from build123d import *

# Parameters (mm, degrees)
BOSS_EXTRUDE1_DEPTH       = 1.5875
F_4_CLEARANCE_HOLE1_D     = 2.9464
F_4_CLEARANCE_HOLE1_DEPTH = 3.302
F_4_CLEARANCE_HOLE1_TIP   = 0.885187864
SKETCH5_W                 = 1.7399
SKETCH5_H                 = 25.4
BOSS_EXTRUDE2_DEPTH       = 1.5875


with BuildPart() as part:
    # Sketch1 → Boss-Extrude1 (new body)
    with BuildSketch(Plane.XY):
        with BuildLine():
            Line((3.58902, 12.7), (3.58902, -12.7))
            ThreePointArc((3.58902, -12.7), (0, -16.28902), (-3.58902, -12.7))
            Line((-3.58902, -12.7), (-3.58902, 12.7))
            ThreePointArc((-3.58902, 12.7), (0, 16.28902), (3.58902, 12.7))
        make_face()
    extrude(amount=BOSS_EXTRUDE1_DEPTH)

    # #4 Clearance Hole1
    with Locations(Plane.XY.offset(1.5875)):
        with Locations((0, 12.7), (0, -12.7)):
            Hole(F_4_CLEARANCE_HOLE1_D / 2, depth=F_4_CLEARANCE_HOLE1_DEPTH)
            with Locations((0, 0, -(F_4_CLEARANCE_HOLE1_DEPTH + F_4_CLEARANCE_HOLE1_TIP / 2))):  # 118° drill point
                Cone(0, F_4_CLEARANCE_HOLE1_D / 2, F_4_CLEARANCE_HOLE1_TIP, mode=Mode.SUBTRACT)

    # Sketch5 → Boss-Extrude2 (add)
    with BuildSketch(Plane.XY.offset(1.5875)):
        with Locations((4.45897, 0)):
            Rectangle(SKETCH5_W, SKETCH5_H)
    extrude(amount=-BOSS_EXTRUDE2_DEPTH)


solid = part.part
For this review, take the finished solid that the model builds, in its own axes (mm). A direction names the side the tool comes from. Round coordinates to 2 decimals unless told otherwise and drop trailing zeros. Order: outer loops, then holes, each group sorted by start corner. A loop starts at its lowest first (then second) coordinate and runs counter-clockwise, first axis right, second up. Notation, with made-up numbers: M 76,-28 L 85,-28 A20 ccw 85,-21 Z; hole C 34.25,71 d3. An arc over 180 degrees is marked long. Write each question's results on one line, items separated by ' | '. Start each with the question number.
1. Clearance check with a flat-ended pin moving along its axis: pin 1 Ø0.8 at (x, z) = (4.5, 1) entering from +Y. State where the tip first meets the part, or that it passes through.
2. Add section B-B (z = 0.45). State the section outline as (x, y) points, then the cut area to 3 significant figures.
3. Add section A-A (x = 0). State the section outline as (y, z) points.
4. Add section C-C (y = 11.5). State the section outline as (x, z) points.
5. Draft analysis for pull direction Y (two halves, no side actions). For faces 3 (the face through (0.19, -11.24, 0.78)), 4 (the face through (4, 12.7, 1)), 5 (the face through (0.08, -16.29, 0.78)), state which applies: pulls with the +Y half, pulls with the -Y half, needs draft (parallel to the pull), parting line crosses it, or undercut.
6. Tool access review of faces 1 (the face through (4, -12.7, 1)), 2 (the face through (-0.08, 16.29, 0.78)): name each direction out of +Z, -Z, +X, -X, +Y, -Y from which nothing blocks a thin tool from reaching the whole face with its end or side.
7. Add section D-D (x = -2.5). State the section outline as (y, z) points.
8. To check wall thickness, follow L1, parallel to Y at x = 0, z = 0.4; L2, parallel to Y at x = 0.5, z = 1.05; L3, parallel to X at y = 12, z = 0.95. State the ranges of each line that lie inside material, in increasing order. Write a range as [from, to].
Output values:
1) pin 1: y = 12.7
2) outline: M -3.59,-12.7 A3.59 ccw 3.59,-12.7 L 5.33,-12.7 L 5.33,12.7 L 3.59,12.7 A3.59 ccw -3.59,12.7 Z; hole C 0,-12.7 d2.95; hole C 0,12.7 d2.95 | area: 253 mm^2
3) outline: M -16.29,0 L -14.17,0 L -14.17,1.59 L -16.29,1.59 Z; M -11.23,0 L 11.23,0 L 11.23,1.59 L -11.23,1.59 Z; M 14.17,0 L 16.29,0 L 16.29,1.59 L 14.17,1.59 Z
4) outline: M -3.59,0 L -0.85,0 L -0.85,1.59 L -3.59,1.59 Z; M 0.85,0 L 5.33,0 L 5.33,1.59 L 0.85,1.59 Z
5) face 3: undercut | face 4: pulls with the +Y half | face 5: pulls with the -Y half
6) face 1: +Z, -Z, +X, -Y | face 2: +Z, -Z, +Y
7) outline: M -15.28,0 L 15.28,0 L 15.28,1.59 L -15.28,1.59 Z
8) L1: [-16.29, -14.17], [-11.23, 11.23], [14.17, 16.29] | L2: [-16.25, -14.09], [-11.31, 11.31], [14.09, 16.25] | L3: [-3.59, -1.3], [1.3, 5.33]
